For this review, take the finished solid that the model builds, in its own axes (mm). A direction names the side the tool comes from. Give positions to 0.01 mm unless a question says otherwise; leave off trailing zeros. Order: outer loops, then holes, each group sorted by start corner. A loop starts at its lowest first (then second) coordinate and runs counter-clockwise, first axis right, second up. Notation, with made-up numbers: (76, -33) - (126, -33) arc R22 cw to (126, -20) - close; hole circle Ø3 at (24.5, 80.25). An arc over 180 degrees is marked (long way). Answer as a JSON object with one key per item and string values. Group by question number.
from build123d import *

# Parameters (mm, degrees)
SKETCH1_R           = 12.5
BOSS_EXTRUDE1_DEPTH = 25
FILLET1_R           = 0.5
SKETCH3_R           = 12.2
BOSS_EXTRUDE2_DEPTH = 30.8
SKETCH4_R           = 3.5
BOSS_EXTRUDE3_DEPTH = 2.5
SKETCH5_R           = 2
BOSS_EXTRUDE4_DEPTH = 9
CUT_EXTRUDE1_START  = -8
CUT_EXTRUDE1_DEPTH  = 8
SKETCH7_R           = 1.5
CUT_EXTRUDE2_DEPTH  = 5
SKETCH8_R           = 7
SKETCH8_W           = 8.453145494
SKETCH8_H           = 4.159745146
BOSS_EXTRUDE5_DEPTH = 5


with BuildPart() as part:
    # Sketch1 → Boss-Extrude1 (new body)
    with BuildSketch(Plane(origin=(0, 0, 0), x_dir=(1, 0, 0), z_dir=(0, 1, 0))):
        with Locations(Location((0, 0, 0), (0, 0, 270))):
            Circle(SKETCH1_R)
    extrude(amount=BOSS_EXTRUDE1_DEPTH)

    # Fillet1
    fillet1_edges = [part.edges().sort_by_distance(p)[0] for p in [
        (0, 0, -12.5),
    ]]
    fillet(fillet1_edges, radius=FILLET1_R)

    # Sketch3 → Boss-Extrude2 (add)
    with BuildSketch(Plane.XZ):
        with Locations(Location((0, 0, 0), (0, 0, 90))):
            Circle(SKETCH3_R)
    extrude(amount=BOSS_EXTRUDE2_DEPTH)

    # Sketch4 → Boss-Extrude3 (add)
    with BuildSketch(Plane(origin=(0, 25, 0), x_dir=(1, 0, 0), z_dir=(0, 1, 0))):
        with Locations(Location((0, 0, 0), (0, 0, 270))):
            Circle(SKETCH4_R)
    extrude(amount=BOSS_EXTRUDE3_DEPTH)

    # Sketch5 → Boss-Extrude4 (add)
    with BuildSketch(Plane(origin=(0, 27.5, 0), x_dir=(1, 0, 0), z_dir=(0, 1, 0))):
        with Locations(Location((0, 0, 0), (0, 0, 270))):
            Circle(SKETCH5_R)
    extrude(amount=BOSS_EXTRUDE4_DEPTH)

    # Sketch6 → Cut-Extrude1 (cut)
    with BuildSketch(Plane(origin=(0, 36.5, 0), x_dir=(1, 0, 0), z_dir=(0, 1, 0)).offset(CUT_EXTRUDE1_START)):
        with BuildLine():
            Line((1.322875656, 1.5), (-1.322875656, 1.5))
            ThreePointArc((-1.322875656, 1.5), (0, 2), (1.322875656, 1.5))
        make_face()
    extrude(amount=CUT_EXTRUDE1_DEPTH, mode=Mode.SUBTRACT)

    # Sketch7 → Cut-Extrude2 (cut)
    with BuildSketch(Plane(origin=(0, 25, 0), x_dir=(1, 0, 0), z_dir=(0, 1, 0))):
        with Locations(Location((-8.5, 0, 0), (0, 0, 270))):
            Circle(SKETCH7_R)
        with Locations(Location((8.5, 0, 0), (0, 0, 270))):
            Circle(SKETCH7_R)
    extrude(amount=-CUT_EXTRUDE2_DEPTH, mode=Mode.SUBTRACT)

    # Sketch8 → Boss-Extrude5 (add)
    with BuildSketch(Plane.XZ.offset(30.8)):
        with Locations(Location((0, 0, 0), (0, 0, 270))):
            Circle(SKETCH8_R)
        with Locations((0, -12.5)):
            Rectangle(SKETCH8_W, SKETCH8_H)
    extrude(amount=BOSS_EXTRUDE5_DEPTH)


solid = part.part
1) For line 1 (X direction, y = 23.55, z = 0); line 2 (Y direction, x = 10.5, z = 3); line 3 (Y direction, x = 4, z = 3.5), list the stretches that pass through material, from the lowest coordinate up.
2) Consider section C-C (y = -4). Give the boundary of the cut face in (x, z), plus the area to 3 significant figures.
3) Mouldability with a two-part tool opening along Z and no side actions: class faces 1 (the face through (7, 23, 0)), 2 (the face through (-3.417, 26.232, -0.759)), 3 (the face through (-3, 25, 3)), 4 (the face through (0, 32, -1.5)) as released by +Z, released by -Z, zero draft, split by the parting line, or undercut.
4) For faces 5 (the face through (-2, 27.5, 2)), 6 (the face through (0, -33, -14.58)), 7 (the face through (-4.227, -33, -13)), 8 (the face through (4.227, -33, -13)), list the 3-axis set-ups (+Z, -Z, +X, -X, +Y, -Y) from which the entire face can be reached by the end or side of a thin tool; tool diameter is ignored.
5) Consider section A-A (x = 0). Give the boundary of the cut face in (y, z), plus the area to 3 significant figures.
6) Consider section B-B (y = 14). Give the boundary of the cut face in (x, z).
7) For pin 1 (1.2 mm diameter, centred on y = -32.5, z = -13, fed in from +X); pin 2 (5 mm diameter, centred on x = 1.5, z = -8, fed in from -Y); pin 3 (2.5 mm diameter, centred on x = 8.5, z = 0, fed in from +Y); pin 4 (6 mm diameter, centred on x = -3, y = 25.5, fed in from -Z), all flat-tipped, find the tip position at first contact; note any pin that passes through.
Result set:
{
 "1": {"line 1": "x = -12.5 to -10, -7 to 7, 10 to 12.5", "line 2": "y = -30.8 to 25", "line 3": "y = -35.8 to 25"},
 "2": {"outline": "circle Ø24.4 at (0, 0)", "area": "468 mm2"},
 "3": {"face 1": "undercut", "face 2": "split by the parting line", "face 3": "zero draft", "face 4": "released by -Z"},
 "4": {"face 5": "+Y", "face 6": "-Z, +X, -X, +Y, -Y", "face 7": "-Z, -X, -Y", "face 8": "-Z, +X, -Y"},
 "5": {"outline": "(-35.8, -14.58) - (-30.8, -14.58) - (-30.8, -12.2) - (0, -12.2) - (0, -12) arc R0.5 ccw to (0.5, -12.5) - (25, -12.5) - (25, -3.5) - (27.5, -3.5) - (27.5, -2) - (28.5, -2) - (28.5, -1.5) - (36.5, -1.5) - (36.5, 2) - (27.5, 2) - (27.5, 3.5) - (25, 3.5) - (25, 12.5) - (0.5, 12.5) arc R0.5 ccw to (0, 12) - (0, 12.2) - (-30.8, 12.2) - (-30.8, 7) - (-35.8, 7) - (-35.8, -7) - (-30.8, -7) - (-30.8, -10.42) - (-35.8, -10.42) - close", "area": "1,520 mm2"},
 "6": {"outline": "circle Ø25 at (0, 0)"},
 "7": {"pin 1": "stops at x = 4.23", "pin 2": "stops at y = -35.8", "pin 3": "stops at y = 20", "pin 4": "stops at z = -12.5"}
}
